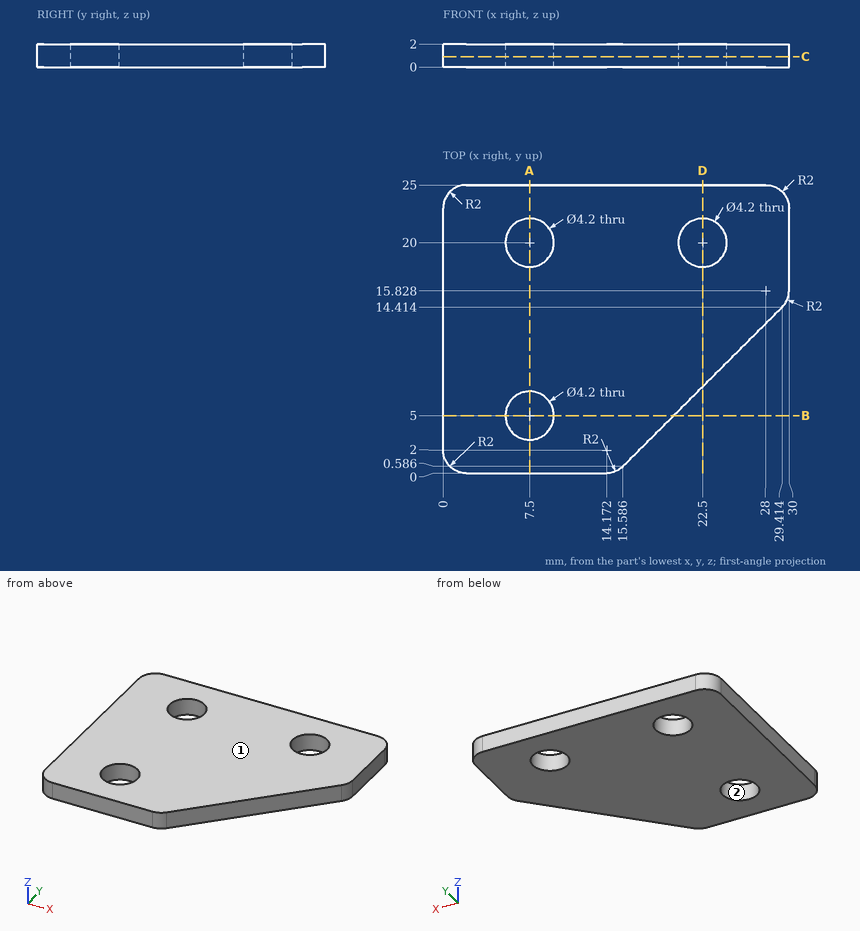
Here's the drawing with two shaded views (mm, measured from the low corner). I have some questions. Coordinates: 2 decimals unless noted, no trailing zeros. Write each loop counter-clockwise with the first axis right and the second up, starting at its lowest first coordinate (ties: lowest second). Pieces come first, ordered by that corner, then holes.
Item 1: If we mould it in two halves opening along Y, with no side actions, what happens to the marked faces 1 and 2? For each: +Y half, -Y half, draft (parallel to the pull), parting line (faces both ways), or undercut.
Item 2: I want a section at A-A on x = 7.5. Write out the boundary of the cut face in (y, z), and give its area (3 significant figures).
Item 3: I want a section at C-C on z = 0.9. Write out the boundary of the cut face in (x, y) (1 decimal).
Item 4: I want a section at D-D on x = 22.5. Write out the boundary of the cut face in (y, z).
Item 5: I want a section at B-B on y = 5. Write out the boundary of the cut face in (x, z).
Item 6: If I drill on line 1 (Y direction, x = 7.5, z = 0.5); line 2 (X direction, y = 5.5, z = 1.8); line 3 (X direction, y = 21.25, z = 1.1), over which ranges is the centre line in solid material (lowest first)?
Findings below:
1. face 1: draft
1. face 2: undercut
2. outline: (0, 0) - (2.9, 0) - (2.9, 2) - (0, 2) - close; (7.1, 0) - (17.9, 0) - (17.9, 2) - (7.1, 2) - close; (22.1, 0) - (25, 0) - (25, 2) - (22.1, 2) - close
2. area: 33.2 mm2
3. outline: (0, 2) arc R2 ccw to (2, 0) - (14.2, 0) arc R2 ccw to (15.6, 0.6) - (29.4, 14.4) arc R2 ccw to (30, 15.8) - (30, 23) arc R2 ccw to (28, 25) - (2, 25) arc R2 ccw to (0, 23) - close; hole circle Ø4.2 at (7.5, 5); hole circle Ø4.2 at (7.5, 20); hole circle Ø4.2 at (22.5, 20)
4. outline: (7.5, 0) - (17.9, 0) - (17.9, 2) - (7.5, 2) - close; (22.1, 0) - (25, 0) - (25, 2) - (22.1, 2) - close
5. outline: (0, 0) - (5.4, 0) - (5.4, 2) - (0, 2) - close; (9.6, 0) - (20, 0) - (20, 2) - (9.6, 2) - close
6. line 1: y = 0 to 2.9, 7.1 to 17.9, 22.1 to 25
6. line 2: x = 0 to 5.46, 9.54 to 20.5
6. line 3: x = 0 to 5.81, 9.19 to 20.81, 24.19 to 30
